Geometry check sheet. Reference: the model listing, model coordinates, mm. Face numbers are marked on the shaded views. A direction names the side the tool comes from. Give positions to 0.01 mm unless a question says otherwise; leave off trailing zeros. Order: outer loops, then holes, each group sorted by start corner. A loop starts at its lowest first (then second) coordinate and runs counter-clockwise, first axis right, second up. Notation, with made-up numbers: M 84,39.5 L 139,39.5 A11 cw 139,57.5 Z; hole C 34,79 d8. An arc over 180 degrees is marked long. Answer as CSV lines item,"result". Start each with the question number.
Q1. Section check A-A, the plane x = 32. Record the boundary of the cut face in (y, z).
Q2. Go/stop test with a flat-tipped pin: pin 1 (5 mm diameter, centred on x = 32, z = 2, fed in from +Y). Record where the tip stops, or that it passes through.
Q3. Thickness scan on line 1 (X direction, y = 7.75, z = 25.8); line 2 (Y direction, x = 32, z = 2.2); line 3 (Y direction, x = 21, z = 20). Record the ranges inside material, lowest first.
Q4. Section check D-D, the plane y = 14.5. Record the boundary of the cut face in (x, z), then the cut area to 3 significant figures.
Q5. Mould release check, pull along X, two halves, no side actions. Record for the marked faces 4, 5, 6 and 7: +X half, -X half, draft (parallel to the pull), parting line (faces both ways), or undercut.
Q6. Set-up check for the marked faces 1, 2 and 3: record each of +Z, -Z, +X, -X, +Y, -Y from which the full face is reachable in a straight line by a thin tool's end or side.
Q7. Section check C-C, the plane z = 28. Record the boundary of the cut face in (x, y).
Q8. Section check B-B, the plane y = 7.75. Record the boundary of the cut face in (x, z), then the cut area to 3 significant figures.
Autodesk Inventor part; units mm, degrees
ref_plane "YZ Plane" through (0, 0, 0) normal (1, 0, 0) x (0, 1, 0)
ref_plane "XZ Plane" through (0, 0, 0) normal (0, 1, 0) x (-1, 0, 0)
ref_plane "XY Plane" through (0, 0, 0) normal (0, 0, 1) x (1, 0, 0)
sketch "Sketch1" plane through (0, 0, 0) normal (0, 0, 1) x (1, 0, 0)
  line L0 (0, 40) -> (5, 40)
  line L1 (5, 40) -> (5, 0)
  line L2 (5, 0) -> (0, 0)
  line L3 (0, 0) -> (0, 40)
  line L4 (5, 0) -> (35, 0)
  line L5 (35, 0) -> (35, 5)
  line L6 (35, 5) -> (5, 5)
  line L7 (5, 5) -> (5, 0)
  line L8 (35, 5) -> (29, 5)
  line L9 (29, 5) -> (29, 10.5)
  line L10 (29, 10.5) -> (35, 10.5)
  line L11 (35, 10.5) -> (35, 5)
  dimension "d0" = 5
  dimension "d1" = 5
  dimension "d2" = 30
  dimension "d4" = 35
  dimension "d7" = 5.5
  dimension "d8" = 6
extrude "Extrusion1" add sketch "Sketch1" along normal blind 30
sketch "Sketch2" plane through (0, 0, 30) normal (0, 0, 1) x (1, 0, 0)
  line L0 (35, 0) -> (35, 10.5)
  line L1 (35, 10.5) -> (29, 10.5)
  line L2 (29, 10.5) -> (29, 5)
  line L3 (29, 5) -> (5, 5)
  line L4 (5, 5) -> (5, 40)
  line L5 (5, 40) -> (0, 40)
  line L6 (0, 40) -> (0, 0)
  line L7 (0, 0) -> (35, 0)
  line L8 (5, 40) -> (9.2143, 10.5)
  line L9 (9.2143, 10.5) -> (8.2143, 10.5)
  line L10 (8.2143, 10.5) -> (5, 33)
  line L11 (5, 5) -> (5, 40)
  line L12 (5, 40) -> (5, 33)
  point P0 (8.7143, 10.5)
  point P1 (32, 10.5)
  dimension "d9" = 1
  dimension "d10" = 7
extrude "Extrusion2" add sketch "Sketch2" against normal up to surface (30 mm away) contours L8 L9 L10 L4
sketch "Sketch3" plane through (0, 0, 30) normal (0, 0, 1) x (1, 0, 0)
  line L0 (35, 0) -> (35, 10.5)
  line L1 (35, 10.5) -> (29, 10.5)
  line L2 (29, 10.5) -> (29, 5)
  line L3 (29, 5) -> (5, 5)
  line L4 (5, 5) -> (5, 33)
  line L5 (5, 33) -> (8.2143, 10.5)
  line L6 (8.2143, 10.5) -> (9.2143, 10.5)
  line L7 (9.2143, 10.5) -> (5, 40)
  line L8 (5, 40) -> (0, 40)
  line L9 (0, 40) -> (0, 0)
  line L10 (0, 0) -> (35, 0)
  point P0 (32, 7.75)
  point P1 (29, 7.75)
  point P2 (32, 10.5)
hole "Hole1" at (32, 7.75, 30) direction (0, 0, -1) diameter 4 end through all
sketch "Sketch4" plane through (29, 10.5, 0) normal (0, 1, 0) x (1, 0, 0)
  line L0 (6, 0) -> (0, 0)
  line L1 (0, 0) -> (0, -30)
  line L2 (6, -30) -> (0, -30)
  line L3 (6, 0) -> (6, -30)
  line L4 (0, 0) -> (0, -30)
  line L5 (6, 0) -> (6, -30)
  line L6 (0, -6) -> (6, -6)
  line L7 (6, -6) -> (6, -24)
  line L8 (6, -24) -> (0, -24)
  line L9 (0, -24) -> (0, -6)
  point P0 (-29, 0)
  dimension "d20" = 6
  dimension "d21" = 6
extrude "Extrusion3" cut sketch "Sketch4" against normal up to surface (5.5 mm away) contours L3 L8 L1 L6
equation "\"d21\" = d20"
properties part number "gpsFrame"
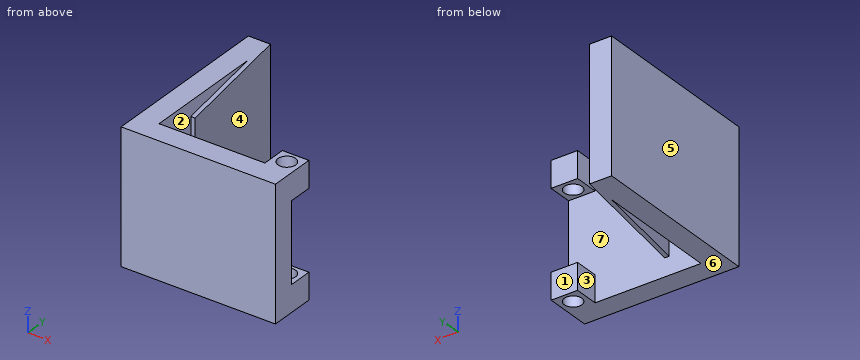
Answer block:
1,outline,"M 0,0 L 5.75,0 L 5.75,6 L 5,6 L 5,24 L 5.75,24 L 5.75,30 L 0,30 Z; M 9.75,0 L 10.5,0 L 10.5,6 L 9.75,6 Z; M 9.75,24 L 10.5,24 L 10.5,30 L 9.75,30 Z"
2,pin 1,"stops at y = 10.5"
3,line 1,"x = 0 to 5, 29 to 30, 34 to 35"
3,line 2,"y = 0 to 5.75, 9.75 to 10.5"
3,line 3,"y = 0 to 5"
4,outline,"M 0,0 L 5,0 L 5,30 L 0,30 Z; M 7.64,0 L 8.64,0 L 8.64,30 L 7.64,30 Z"
4,area,"180 mm2"
5,face 4,"+X half"
5,face 5,"-X half"
5,face 6,"draft"
5,face 7,"undercut"
6,face 1,"+Z, -Z, +X, +Y"
6,face 2,"+Z, -Z"
6,face 3,"+Z, -Z, +Y"
7,outline,"M 0,0 L 35,0 L 35,10.5 L 29,10.5 L 29,5 L 5,5 L 5,33 L 8.21,10.5 L 9.21,10.5 L 5,40 L 0,40 Z; hole C 32,7.75 d4"
8,outline,"M 0,0 L 5,0 L 5,30 L 0,30 Z; M 29,0 L 30,0 L 30,6 L 29,6 Z; M 29,24 L 30,24 L 30,30 L 29,30 Z; M 34,0 L 35,0 L 35,6 L 34,6 Z; M 34,24 L 35,24 L 35,30 L 34,30 Z"
8,area,"174 mm2"
